```python
from build123d import *

# Parameters (mm, degrees)
ESBO_O1_W                = 35
ESBO_O1_H                = 13
RESSALTO_EXTRUS_O1_DEPTH = 1.5
ESBO_O2_W                = 22
ESBO_O2_H                = 13
RESSALTO_EXTRUS_O2_DEPTH = 8.5
ESBO_O3_W                = 20
ESBO_O3_H                = 9.770333273
CORTE_EXTRUS_O1_DEPTH    = 2.5
ESBO_O4_R                = 1.5
CORTE_EXTRUS_O2_DEPTH    = 2.5


with BuildPart() as part:
    # Esboço1 → Ressalto-extrusão1 (new body)
    with BuildSketch(Plane.XY):
        with Locations((17.5, 6.5)):
            Rectangle(ESBO_O1_W, ESBO_O1_H)
    extrude(amount=RESSALTO_EXTRUS_O1_DEPTH)

    # Esboço2 → Ressalto-extrusão2 (add)
    with BuildSketch(Plane.XY.offset(1.5)):
        with Locations((17.5, 6.5)):
            Rectangle(ESBO_O2_W, ESBO_O2_H)
    extrude(amount=RESSALTO_EXTRUS_O2_DEPTH)

    # Esboço3 → Corte-extrusão1 (cut)
    with BuildSketch(Plane(origin=(0, 0, 0), x_dir=(-1, 0, 0), z_dir=(0, 0, -1))):
        with Locations((-17.5, 6.364833363)):
            Rectangle(ESBO_O3_W, ESBO_O3_H)
    extrude(amount=-CORTE_EXTRUS_O1_DEPTH, mode=Mode.SUBTRACT)

    # Esboço4 → Corte-extrusão2 (cut)
    with BuildSketch(Plane(origin=(0, 0, 0), x_dir=(-1, 0, 0), z_dir=(0, 0, -1))):
        with Locations((-32.5, 6.5)):
            Circle(ESBO_O4_R)
        with Locations((-2.5, 6.5)):
            Circle(ESBO_O4_R)
    extrude(amount=-CORTE_EXTRUS_O2_DEPTH, mode=Mode.SUBTRACT)


solid = part.part
```
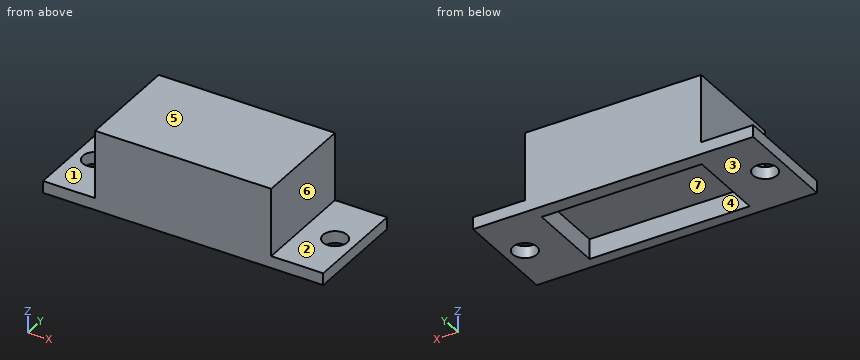
The listing builds one solid part. Answer for the finished solid, in the listing's coordinates (mm). Face numbers are marked on the shaded views. A direction names the side the tool comes from. Coordinates: 2 decimals unless noted, no trailing zeros. Write each loop counter-clockwise with the first axis right and the second up, starting at its lowest first coordinate (ties: lowest second). Pieces come first, ordered by that corner, then holes. Notation, with made-up numbers: (9.5, 57.5) - (14.5, 57.5) arc R17 ccw to (14.5, 88.5) - close; hole circle Ø9 at (-10, 50.5). An arc over 180 degrees is marked (long way). One line per item, written item: value.
1) Each of these flat-tipped pins is pushed along its axis until it touches: pin 1 Ø4 at (y, z) = (3.5, 9) entering from -X; pin 2 Ø2 at (x, y) = (2, 6) entering from +Z; pin 3 Ø4 at (y, z) = (8, 5.5) entering from +X; pin 4 Ø2.5 at (x, y) = (32.5, 6.5) entering from -Z. Where does it stop, or does it pass through?
Geometry check:
pin 1: stops at x = 6.5
pin 2: stops at z = 1.5
pin 3: stops at x = 28.5
pin 4: passes through
2) Consider line 1 along Y through (x, z) = (32.5, 0.6); line 2 along Y through (x, z) = (25.5, 1.75); line 3 along X through (y, z) = (5.75, 2.25). Determine where each line is inside the solid, lowest interval first. Write a range as from..to.
Geometry check:
line 1: y = 0..5, 8..13
line 2: y = 0..1.48, 11.25..13
line 3: x = 6.5..7.5, 27.5..28.5
3) Find section C-C (z = 1). Give the vertices of the cut face in (x, y), and give its area (3 significant figures).
Geometry check:
outline: (0, 0) - (35, 0) - (35, 13) - (0, 13) - close; hole circle Ø3 at (2.5, 6.5); hole (7.5, 1.48) - (27.5, 1.48) - (27.5, 11.25) - (7.5, 11.25) - close; hole circle Ø3 at (32.5, 6.5)
area: 245 mm2
4) A tool of negligible diameter and unlimited length cuts with its end or side. For the marked faces 1, 2 and 3, from which of +Z, -Z, +X, -X, +Y, -Y can it reach the whole face along a straight path? Write none if from no direction.
Geometry check:
face 1: +Z, -X, +Y, -Y
face 2: +Z, +X, +Y, -Y
face 3: -Z, +X, -X, +Y, -Y
5) Find section A-A (y = 6.5). Give the vertices of the cut face in (x, z).
Geometry check:
outline: (0, 0) - (1, 0) - (1, 1.5) - (0, 1.5) - close; (4, 0) - (7.5, 0) - (7.5, 2.5) - (27.5, 2.5) - (27.5, 0) - (31, 0) - (31, 1.5) - (28.5, 1.5) - (28.5, 10) - (6.5, 10) - (6.5, 1.5) - (4, 1.5) - close; (34, 0) - (35, 0) - (35, 1.5) - (34, 1.5) - close
6) For a pull along X with two mould halves and no side action, classify the marked faces 4, 5, 6 and 7 as pulls with the +X half, pulls with the -X half, needs draft (parallel to the pull), parting line crosses it, or undercut.
Geometry check:
face 4: undercut
face 5: needs draft
face 6: pulls with the +X half
face 7: undercut
7) Find section D-D (y = 10.25). Give the vertices of the cut face in (x, z).
Geometry check:
outline: (0, 0) - (7.5, 0) - (7.5, 2.5) - (27.5, 2.5) - (27.5, 0) - (35, 0) - (35, 1.5) - (28.5, 1.5) - (28.5, 10) - (6.5, 10) - (6.5, 1.5) - (0, 1.5) - close
8) Find section B-B (x = 32.5). Give the vertices of the cut face in (y, z).
Geometry check:
outline: (0, 0) - (5, 0) - (5, 1.5) - (0, 1.5) - close; (8, 0) - (13, 0) - (13, 1.5) - (8, 1.5) - close
